Source: CAD feature listing. Evaluate the final solid. Frame: model axes, mm. Face numbers are marked on the shaded views. A direction names the side the tool comes from. Coordinates: 2 decimals unless noted, no trailing zeros. Loops run counter-clockwise (first coordinate to the right, second up) from the corner with the lowest first, then second, coordinate; pieces in that order, holes last. Notation, with made-up numbers: (-6, -35) - (50, -35) arc R32 ccw to (50, 0) - close; hole circle Ø11 at (55, 42). An arc over 180 degrees is marked (long way). Write item = value, one per line. Start each with the question number.
from build123d import *

# Parameters (mm, degrees)
F1_DEPTH = 15.24
F2_R     = 5.08
F3_R     = 5.08
F4_DEPTH = 16.764


with BuildPart() as f1:
    # F0 (on Top) → F1 (new body)
    with BuildSketch(Plane.XY):
        Polygon((0, -19.558), (16.937725, -9.779), (16.937725, 9.779), (0, 19.558), (-16.937725, 9.779), (-16.937725, -9.779), align=None)
    extrude(amount=F1_DEPTH)

    # F2
    f2_edges = [f1.edges().sort_by_distance(p)[0] for p in [
        (-8.468862, -14.6685, 15.24),
        (8.468862, -14.6685, 15.24),
        (16.937725, 0, 15.24),
        (8.468862, 14.6685, 15.24),
        (-8.468862, 14.6685, 15.24),
        (-16.937725, 0, 15.24),
    ]]
    fillet(f2_edges, radius=F2_R)

    # F3
    f3_edges = [f1.edges().sort_by_distance(p)[0] for p in [
        (-8.468862, -14.6685, 0),
        (8.468862, -14.6685, 0),
        (16.937725, 0, 0),
        (8.468862, 14.6685, 0),
        (-8.468862, 14.6685, 0),
        (-16.937725, 0, 0),
    ]]
    fillet(f3_edges, radius=F3_R)

    # F0 (on Top) → F4 (join)
    with BuildSketch(Plane.XY):
        with BuildLine():
            Line((-38.527725, -47.173977), (-16.937725, -9.779))
            Line((-16.937725, -9.779), (-16.937725, 9.779))
            Line((-16.937725, 9.779), (-38.527725, 47.173977))
            Line((-38.527725, 47.173977), (-60.727019, 9.779))
            Line((-60.727019, 9.779), (-60.727019, 7.295595))
            ThreePointArc((-60.727019, 7.295595), (-59.776888, 3.702654), (-59.457019, 0))
            ThreePointArc((-59.457019, 0), (-59.776888, -3.702654), (-60.727019, -7.295595))
            Line((-60.727019, -7.295595), (-60.727019, -9.779))
            Line((-60.727019, -9.779), (-38.527725, -47.173977))
        make_face()
        with BuildLine():
            Line((-16.937725, 9.779), (0, 19.558))
            Line((0, 19.558), (-21.59, 56.952977))
            Line((-21.59, 56.952977), (-23.740692, 55.711274))
            ThreePointArc((-23.740692, 55.711274), (-29.423862, 50.963625), (-36.377033, 48.41568))
            Line((-36.377033, 48.41568), (-38.527725, 47.173977))
            Line((-38.527725, 47.173977), (-16.937725, 9.779))
        make_face()
        Polygon((-21.59, 56.952977), (0, 19.558), (21.59, 56.952977), align=None)
        Polygon((16.937725, 9.779), (16.937725, -9.779), (38.527725, -47.173977), (60.727019, -9.779), (17.55615, -9.779), (17.55615, 9.779), (60.727019, 9.779), (38.527725, 47.173977), align=None)
        with BuildLine():
            Line((0, 19.558), (16.937725, 9.779))
            Line((16.937725, 9.779), (38.527725, 47.173977))
            Line((38.527725, 47.173977), (36.377033, 48.41568))
            ThreePointArc((36.377033, 48.41568), (29.423862, 50.963625), (23.740692, 55.711274))
            Line((23.740692, 55.711274), (21.59, 56.952977))
            Line((21.59, 56.952977), (0, 19.558))
        make_face()
        with BuildLine():
            Line((17.55615, -9.779), (60.727019, -9.779))
            Line((60.727019, -9.779), (60.727019, -7.295595))
            ThreePointArc((60.727019, -7.295595), (59.457019, 0), (60.727019, 7.295595))
            Line((60.727019, 7.295595), (60.727019, 9.779))
            Line((60.727019, 9.779), (17.55615, 9.779))
            Line((17.55615, 9.779), (17.55615, -9.779))
        make_face()
        with BuildLine():
            Line((38.527725, -47.173977), (16.937725, -9.779))
            Line((16.937725, -9.779), (0, -19.558))
            Line((0, -19.558), (21.59, -56.952977))
            Line((21.59, -56.952977), (23.740692, -55.711274))
            ThreePointArc((23.740692, -55.711274), (29.423862, -50.963625), (36.377033, -48.41568))
            Line((36.377033, -48.41568), (38.527725, -47.173977))
        make_face()
        Polygon((21.59, -56.952977), (0, -19.558), (-21.59, -56.952977), align=None)
        with BuildLine():
            Line((-21.59, -56.952977), (0, -19.558))
            Line((0, -19.558), (-16.937725, -9.779))
            Line((-16.937725, -9.779), (-38.527725, -47.173977))
            Line((-38.527725, -47.173977), (-36.377033, -48.41568))
            ThreePointArc((-36.377033, -48.41568), (-29.423862, -50.963625), (-23.740692, -55.711274))
            Line((-23.740692, -55.711274), (-21.59, -56.952977))
        make_face()
    extrude(amount=F4_DEPTH)


solid = f1.part
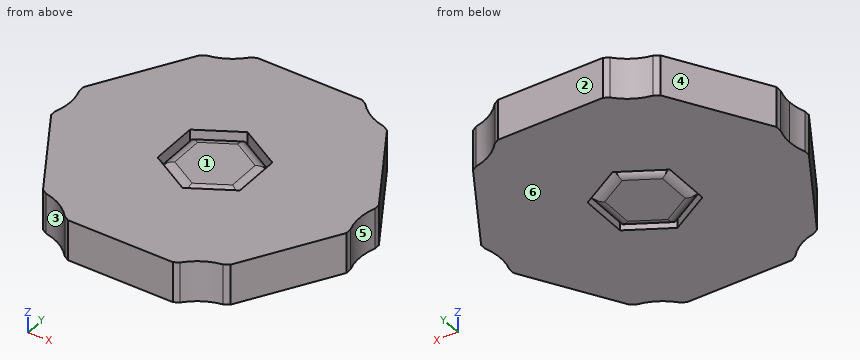
Item 1: Material intervals for L1, parallel to Y at x = -3, z = 3.25; L2, parallel to X at y = 18, z = 3.75; L3, parallel to Y at x = -1.5, z = 2.75, sorted ascending. Write a range as [from, to].
Item 2: Reachability of the marked faces 1 and 2 from +Z, -Z, +X, -X, +Y, -Y: full face, straight path, thin tool, end or side. Return the list, or none.
Item 3: Cut plane C-C (x = -43.5). Return the cut outline in (y, z), then the cut area to 3 significant figures.
Item 4: Draft query along Y for the marked faces 3, 4, 5 and 6. Return one class per face: released by +Y, released by -Y, zero draft, split by the parting line, or undercut.
Item 5: Cut plane D-D (y = 34). Return the cut outline in (x, z), then the cut area to 3 significant figures.
Item 6: Cut plane B-B (z = 2). State how many separate pieces and enclosed holes the cut face has, then the cut area to 3 significant figures.
Item 7: Cut plane A-A (z = 8.5). Return the cut outline in (x, y), then the cut area to 3 significant figures.
Item 8: First-contact query: pin 1 (3 mm diameter, centred on x = -31.5, y = 1, fed in from -Z); pin 2 (3.5 mm diameter, centred on y = -2, z = 14, fed in from +X); pin 3 (3 mm diameter, centred on x = -43.5, z = 8.5, fed in from +Y); pin 4 (3 mm diameter, centred on y = -17, z = 4.5, fed in from -X). Flat tips, straight axial feed; report the tip coordinate or a pass-through.
Responses:
q1.L1 = [-56.95, -17.83], [-17.43, 17.43], [17.83, 56.95]
q1.L2 = [-55.85, -2.7], [-2.34, 2.34], [2.7, 55.85]
q1.L3 = [-56.95, -18.69], [-18.04, 18.04], [18.69, 56.95]
q2.face_1 = +Z
q2.face_2 = +Z, -Z, +X, -X, +Y
q3.outline = (-38.8, 0) - (38.8, 0) - (38.8, 16.76) - (-38.8, 16.76) - close
q3.area = 1,300 mm2
q4.face_3 = released by -Y
q4.face_4 = released by +Y
q4.face_5 = undercut
q4.face_6 = zero draft
q5.outline = (-46.35, 0) - (46.35, 0) - (46.35, 16.76) - (-46.35, 16.76) - close
q5.area = 1,550 mm2
q6.separate_pieces = 2
q6.enclosed_holes = 1
q6.area = 10,800 mm2
q7.outline = (-60.73, -9.78) - (-38.53, -47.17) - (-36.38, -48.42) arc R21.59 cw to (-23.74, -55.71) - (-21.59, -56.95) - (21.59, -56.95) - (23.74, -55.71) arc R21.59 cw to (36.38, -48.42) - (38.53, -47.17) - (60.73, -9.78) - (60.73, -7.3) arc R21.59 cw to (60.73, 7.3) - (60.73, 9.78) - (38.53, 47.17) - (36.38, 48.42) arc R21.59 cw to (23.74, 55.71) - (21.59, 56.95) - (-21.59, 56.95) - (-23.74, 55.71) arc R21.59 cw to (-36.38, 48.42) - (-38.53, 47.17) - (-60.73, 9.78) - (-60.73, 7.3) arc R21.59 cw to (-59.46, 0) arc R21.59 cw to (-60.73, -7.3) - close
q7.area = 10,900 mm2
q8.pin_1 = 0
q8.pin_2 = 59.79
q8.pin_3 = 41.32
q8.pin_4 = -57.33
